from build123d import *

# Parameters (mm, degrees)
BOSS_EXTRUDE2_DEPTH = 5
SKETCH3_W           = 5
SKETCH3_H           = 40
CUT_EXTRUDE1_DEPTH  = 5
SKETCH4_R           = 1.5875
CUT_EXTRUDE2_DEPTH  = 6


with BuildPart() as part:
    # Sketch2 → Boss-Extrude2 (new body)
    with BuildSketch(Plane.XY):
        Polygon((-7.5, 40), (7.5, 40), (7.5, 35), (27.5, 35), (27.5, -35), (7.5, -35), (7.5, -40), (-7.5, -40), (-7.5, -35), (-27.5, -35), (-27.5, 35), (-7.5, 35), align=None)
    extrude(amount=BOSS_EXTRUDE2_DEPTH)

    # Sketch3 → Cut-Extrude1 (cut)
    with BuildSketch(Plane.XY.offset(5)):
        with Locations((-25, 0)):
            Rectangle(SKETCH3_W, SKETCH3_H)
    cut_extrude1 = extrude(amount=-CUT_EXTRUDE1_DEPTH, mode=Mode.SUBTRACT)

    # Mirror1: Cut-Extrude1 across plane
    add(cut_extrude1.mirror(Plane(origin=(0, 0, 0), x_dir=(0, 0, 1), z_dir=(1, 0, 0))), mode=Mode.SUBTRACT)

    # Sketch4 → Cut-Extrude2 (cut, through all)
    with BuildSketch(Plane.XY.offset(5)):
        with Locations((-22.5, 20)):
            Circle(SKETCH4_R)
        with Locations((-7.5, 35)):
            Circle(SKETCH4_R)
        with Locations((7.5, 35)):
            Circle(SKETCH4_R)
        with Locations((22.5, 20)):
            Circle(SKETCH4_R)
        with Locations((22.5, -20)):
            Circle(SKETCH4_R)
        with Locations((7.5, -35)):
            Circle(SKETCH4_R)
        with Locations((-7.5, -35)):
            Circle(SKETCH4_R)
        with Locations((-22.5, -20)):
            Circle(SKETCH4_R)
    extrude(amount=-CUT_EXTRUDE2_DEPTH, mode=Mode.SUBTRACT)


solid = part.part
Source: CAD feature listing. Evaluate the final solid. Frame: model axes, mm. A direction names the side the tool comes from. Give positions to 0.01 mm unless a question says otherwise; leave off trailing zeros. Write each loop counter-clockwise with the first axis right and the second up, starting at its lowest first coordinate (ties: lowest second). Pieces come first, ordered by that corner, then holes. Notation, with made-up numbers: (29, 14.5) - (49, 14.5) arc R26 cw to (49, 40.5) - close; hole circle Ø2 at (8, -35.5). An arc over 180 degrees is marked (long way). Write item = value, one per line. Start each with the question number.
Q1. Pin query (flat end, axial travel): pin 1 Ø1 at (x, z) = (-26, 2.5) entering from +Y; pin 2 Ø1.9 at (x, y) = (-22.5, -20) entering from +Z; pin 3 Ø1.7 at (y, z) = (39, 2.5) entering from +X; pin 4 Ø1.5 at (y, z) = (7, 2.5) entering from -X. Return the tip coordinate at first contact, or that it passes through.
Q2. Reachability of faces 1 (the flat face through (18, 35, 2)), 2 (the cylindrical face through (21.341, -21.085, 2.535)), 3 (the flat face through (-7.5, 38, 2)), 4 (the flat face through (-7.5, -38, 2)), 5 (the flat face through (26, -20, 3)) from +Z, -Z, +X, -X, +Y, -Y: full face, straight path, thin tool, end or side. Return the list, or none.
Q3. Material intervals for probe 1 along Y at (x, z) = (-22, 4.35); probe 2 along Y at (x, z) = (14.5, 3.15); probe 3 along X at (y, z) = (17, 3.9), sorted ascending.
Q4. Draft query along Y for faces 6 (the flat face through (-18, 35, 2)), 7 (the flat face through (27.5, 28, 2)), 8 (the cylindrical face through (-6.341, -33.915, 2.535)), 9 (the flat face through (0, -40, 2)). Return one class per face: +Y half, -Y half, draft (parallel to the pull), parting line (faces both ways), or undercut.
Q5. Cut plane B-B, the plane y = 14. Return loops of the section in (x, z).
Q6. Cut plane A-A, the plane z = 2.45. Return loops of the section in (x, y) (1 decimal).
Computed values:
q1.pin_1 = 35
q1.pin_2 = through
q1.pin_3 = 7.5
q1.pin_4 = -22.5
q2.face_1 = +Z, -Z, +X, +Y
q2.face_2 = +Z, -Z
q2.face_3 = +Z, -Z, -X, +Y
q2.face_4 = +Z, -Z, -X, -Y
q2.face_5 = +Z, -Z, +X
q3.probe_1 = -35 to -21.51, -18.49 to 18.49, 21.51 to 35
q3.probe_2 = -35 to 35
q3.probe_3 = -22.5 to 22.5
q4.face_6 = +Y half
q4.face_7 = draft
q4.face_8 = undercut
q4.face_9 = -Y half
q5.outline = (-22.5, 0) - (22.5, 0) - (22.5, 5) - (-22.5, 5) - close
q6.outline = (-27.5, -35) - (-9.1, -35) arc R1.6 cw (long way) to (-7.5, -36.6) - (-7.5, -40) - (7.5, -40) - (7.5, -36.6) arc R1.6 cw (long way) to (9.1, -35) - (27.5, -35) - (27.5, -20) - (24.1, -20) arc R1.6 cw (long way) to (22.5, -18.4) - (22.5, 18.4) arc R1.6 cw (long way) to (24.1, 20) - (27.5, 20) - (27.5, 35) - (9.1, 35) arc R1.6 cw (long way) to (7.5, 36.6) - (7.5, 40) - (-7.5, 40) - (-7.5, 36.6) arc R1.6 cw (long way) to (-9.1, 35) - (-27.5, 35) - (-27.5, 20) - (-24.1, 20) arc R1.6 cw (long way) to (-22.5, 18.4) - (-22.5, -18.4) arc R1.6 cw (long way) to (-24.1, -20) - (-27.5, -20) - close
